Geometry: final body of the model. Coordinates: model frame, mm. A direction names the side the tool comes from. Give positions to 0.01 mm unless a question says otherwise; leave off trailing zeros. Order: outer loops, then holes, each group sorted by start corner. A loop starts at its lowest first (then second) coordinate and runs counter-clockwise, first axis right, second up. Notation, with made-up numbers: (9.25, 78.25) - (34.25, 78.25) arc R9 ccw to (34.25, 86.25) - close; hole circle Ø11 at (14, 10). An arc over 180 degrees is marked (long way). One line per item, written item: value.
```python
from build123d import *

# Parameters (mm, degrees)
ESQUISSE2_R             = 2.5
BASE_EXTRUSION_DEPTH    = 7
CHANFREIN1_SIZE         = 0.5
ENL_V_MAT_EXTRU_1_DEPTH = 2.25


with BuildPart() as part:
    # Esquisse2 → Base-Extrusion (new body)
    with BuildSketch(Plane(origin=(0, 0, 0), x_dir=(1, 0, 0), z_dir=(0, 1, 0))):
        with Locations(Location((0, 0, 0), (0, 0, 270))):  # turned: the seam where the file's is
            Circle(ESQUISSE2_R)
    extrude(amount=-BASE_EXTRUSION_DEPTH)

    # Chanfrein1
    chanfrein1_edges = [part.edges().sort_by_distance(p)[0] for p in [
        (0, -7, -2.5),
    ]]
    chamfer(chanfrein1_edges, length=CHANFREIN1_SIZE)

    # Esquisse5 → Boss.-Révol.1 (revolve)
    with BuildSketch(Plane.XY, mode=Mode.PRIVATE) as boss_r_vol_1_sk:
        with BuildLine():
            Line((2, 4.5), (2, 2.25))
            Line((2, 2.25), (0, 1.095299462))
            Line((0, 1.095299462), (0, 0))
            Line((0, 0), (4.25, 0))
            Line((4.25, 0), (4.25, 4.05))
            ThreePointArc((4.25, 4.05), (4.118198052, 4.368198052), (3.8, 4.5))
            Line((3.8, 4.5), (2, 4.5))
        make_face()
    revolve(boss_r_vol_1_sk.sketch.rotate(Axis((0, 4.5, 0), (0, -1, 0)), 90), axis=Axis((0, 4.5, 0), (0, -1, 0)))  # turned: the seam where the file's is

    # Esquisse7 → Enlèv. mat.-Extru.1 (cut)
    with BuildSketch(Plane(origin=(0, 4.5, 0), x_dir=(-1, 0, 0), z_dir=(0, 1, 0))):
        Polygon((1.154700538, 2), (-1.154700538, 2), (-2.309401077, 0), (-1.154700538, -2), (1.154700538, -2), (2.309401077, 0), align=None)
    extrude(amount=-ENL_V_MAT_EXTRU_1_DEPTH, mode=Mode.SUBTRACT)


solid = part.part
```
1) Mould query, pull axis Z, two halves, no side actions, for faces 4 (the face through (0, 3, -2)), 5 (the face through (0, -7, 0)), 6 (the face through (-2.44, -3.2, -0.54)). Classes: released by +Z, released by -Z, zero draft, split by the parting line, or undercut.
Answers below:
face 4: undercut
face 5: zero draft
face 6: split by the parting line
2) Material intervals for line 1 along Z through (x, y) = (-1.5, -1); line 2 along X through (y, z) = (3, -0.75); line 3 along Z through (x, y) = (0.75, 3.25), sorted ascending.
Answers below:
line 1: -2 to 2
line 2: -4.18 to -1.88, 1.88 to 4.18
line 3: -4.18 to -2, 2 to 4.18
3) Section B-B, the plane y = 2. Return loops of the section in (x, z).
Answers below:
outline: circle Ø8.5 at (0, 0); hole circle Ø3.13 at (0, 0)
4) Section A-A, the plane y = 0.75. Return loops of the section in (x, z), then the cut area to 3 significant figures.
Answers below:
outline: circle Ø8.5 at (0, 0)
area: 56.7 mm^2
5) First-contact query: pin 1 (2 mm diameter, centred on y = 0.5, z = -2, fed in from +X); pin 2 (1.5 mm diameter, centred on x = 2.5, y = 2, fed in from -Z); pin 3 (0.7 mm diameter, centred on x = 0.5, y = 3.5, fed in from -Z). Flat tips, straight axial feed; report the tip coordinate or a pass-through.
Answers below:
pin 1: x = 4.13
pin 2: z = -3.87
pin 3: z = -4.25
6) Set-up query: faces 1 (the face through (0, 3, 2)), 2 (the face through (2, 0, -2)), 3 (the face through (-4.214, 2.053, -0.553)). Return all of +Z, -Z, +X, -X, +Y, -Y with unobstructed straight access to the full face (end or side cutting, diameter ignored); none if empty.
Answers below:
face 1: +Y
face 2: -Y
face 3: +Y, -Y
